Read the model definition and answer for the solid it produces. Units are mm, in the model's axes. A direction names the side the tool comes from. Coordinates: 2 decimals unless noted, no trailing zeros. Order: outer loops, then holes, each group sorted by start corner. A loop starts at its lowest first (then second) coordinate and runs counter-clockwise, first axis right, second up.
```python
from build123d import *

# Parameters (mm, degrees)
SKETCH1_W           = 42
SKETCH1_H           = 67.5
SKETCH1_R           = 3
SKETCH1_R_2         = 2.25
BOSS_EXTRUDE1_DEPTH = 4
SKETCH2_W           = 42
SKETCH2_H           = 3
BOSS_EXTRUDE2_DEPTH = 12
SKETCH3_W           = 42
SKETCH3_H           = 16
SKETCH3_R           = 3
BOSS_EXTRUDE3_DEPTH = 3
CUT_EXTRUDE1_REACH  = 74.479
SKETCH4_R           = 1.6
FILLET1_R           = 4
SKETCH5_W           = 16
SKETCH5_H           = 16
BOSS_EXTRUDE4_DEPTH = 3
FILLET3_R           = 2
FILLET4_R           = 2


with BuildPart() as part:
    # Sketch1 → Boss-Extrude1 (new body)
    with BuildSketch(Plane.XY):
        Rectangle(SKETCH1_W, SKETCH1_H)
        with Locations((-7.5, -24.75)):
            Circle(SKETCH1_R, mode=Mode.SUBTRACT)
        with Locations((1.5, 29.25)):
            Circle(SKETCH1_R_2, mode=Mode.SUBTRACT)
        with Locations((-16.5, 29.25)):
            Circle(SKETCH1_R_2, mode=Mode.SUBTRACT)
        with Locations((1.5, 5.25)):
            Circle(SKETCH1_R_2, mode=Mode.SUBTRACT)
        with Locations((-16.5, 5.25)):
            Circle(SKETCH1_R_2, mode=Mode.SUBTRACT)
    extrude(amount=BOSS_EXTRUDE1_DEPTH)

    # Sketch2 → Boss-Extrude2 (add)
    with BuildSketch(Plane.XY.offset(4)):
        with Locations((0, -32.25)):
            Rectangle(SKETCH2_W, SKETCH2_H)
    extrude(amount=BOSS_EXTRUDE2_DEPTH)

    # Sketch3 → Boss-Extrude3 (add)
    with BuildSketch(Plane.XY.offset(4)):
        with Locations((0, -22.75)):
            Rectangle(SKETCH3_W, SKETCH3_H)
        with Locations((-7.5, -24.75)):
            Circle(SKETCH3_R, mode=Mode.SUBTRACT)
    extrude(amount=BOSS_EXTRUDE3_DEPTH)

    # Sketch4 → Cut-Extrude1 (cut, up to next)
    with BuildSketch(Plane.XZ.offset(33.75), mode=Mode.PRIVATE) as cut_extrude1_sk1:
        with Locations(Location((-15.5, 12.5, 0), (0, 0, 270))):
            Circle(SKETCH4_R)
    cut_extrude1_tool1 = extrude(cut_extrude1_sk1.sketch, amount=-CUT_EXTRUDE1_REACH, mode=Mode.PRIVATE) & part.part
    # Sketch4 → Cut-Extrude1 (cut, up to next)
    with BuildSketch(Plane.XZ.offset(33.75), mode=Mode.PRIVATE) as cut_extrude1_sk2:
        with Locations(Location((15.285724533, 12.5, 0), (0, 0, 270))):
            Circle(SKETCH4_R)
    cut_extrude1_tool2 = extrude(cut_extrude1_sk2.sketch, amount=-CUT_EXTRUDE1_REACH, mode=Mode.PRIVATE) & part.part
    add(cut_extrude1_tool1.solids().sort_by_distance((-15.5, -33.75, 12.5))[0], mode=Mode.SUBTRACT)
    add(cut_extrude1_tool2.solids().sort_by_distance((15.285725, -33.75, 12.5))[0], mode=Mode.SUBTRACT)

    # Fillet1
    # the kernel refuses this fillet: 4 mm, written as the material it adds along each edge
    with BuildSketch(Plane(origin=(-21, -14.75, 4), x_dir=(0, 1, 0), z_dir=(1, 0, 0))) as fillet1_piece_1:
        with BuildLine():
            CenterArc((3.872983346, 4), FILLET1_R, 194.477512186, 75.522487814)
            Line((0, 3), (0, 0))
            Line((0, 0), (3.872983346, 0))
        make_face()
    extrude(amount=42)
    # the kernel refuses this fillet: 4 mm, written as the material it takes off along each edge
    with BuildSketch(Plane(origin=(21, -20.75, 16), x_dir=(0, 0, -1), z_dir=(0, -1, 0)), Plane(origin=(-21, -43.75, 16), x_dir=(0, 0, -1), z_dir=(0, 1, 0))) as fillet1_2_piece_1:
        with BuildLine():
            CenterArc((FILLET1_R, -FILLET1_R), FILLET1_R, 90, 90)
            Line((0, -FILLET1_R), (0, 0))
            Line((0, 0), (FILLET1_R, 0))
        make_face()
    extrude(amount=23, mode=Mode.SUBTRACT)
    with BuildSketch(Plane(origin=(21, 33.75, -10), x_dir=(-1, 0, 0), z_dir=(0, 0, 1))) as fillet1_2_piece_2:
        with BuildLine():
            CenterArc((FILLET1_R, FILLET1_R), FILLET1_R, 180, 90)
            Line((0, FILLET1_R), (0, 0))
            Line((0, 0), (FILLET1_R, 0))
        make_face()
    extrude(amount=24, mode=Mode.SUBTRACT)
    with BuildSketch(Plane(origin=(-21, 33.75, -10), x_dir=(1, 0, 0), z_dir=(0, 0, 1))) as fillet1_2_piece_3:
        with BuildLine():
            CenterArc((FILLET1_R, -FILLET1_R), FILLET1_R, 90, 90)
            Line((0, -FILLET1_R), (0, 0))
            Line((0, 0), (FILLET1_R, 0))
        make_face()
    extrude(amount=24, mode=Mode.SUBTRACT)

    # Sketch5 → Boss-Extrude4 (add)
    with BuildSketch(Plane.XZ.offset(33.75)):
        with Locations((-0.071835854, 8)):
            Rectangle(SKETCH5_W, SKETCH5_H)
    extrude(amount=BOSS_EXTRUDE4_DEPTH)

    # Fillet3
    fillet3_edges = [part.edges().sort_by_distance(p)[0] for p in [
        (-8.071835854, -33.75, 8),
        (7.928164146, -33.75, 8),
    ]]
    fillet(fillet3_edges, radius=FILLET3_R)

    # Fillet4
    fillet4_edges = [part.edges().sort_by_distance(p)[0] for p in [
        (7.928164146, -36.75, 8),
        (-8.071835854, -36.75, 8),
    ]]
    fillet(fillet4_edges, radius=FILLET4_R)


solid = part.part
```
1) A cutting plane is placed at B-B, the plane y = 5.25. Determine the outline of the cut face in (x, z).
A:
outline: (-21, 0) - (-18.75, 0) - (-18.75, 4) - (-21, 4) - close; (-14.25, 0) - (-0.75, 0) - (-0.75, 4) - (-14.25, 4) - close; (3.75, 0) - (21, 0) - (21, 4) - (3.75, 4) - close
2) Straight lines are drawn through the part: line 1 (Y direction, x = 1.5, z = 1.2); line 2 (Y direction, x = -16.5, z = 2.4); line 3 (X direction, y = -32, z = 12.5). For each, find the intervals that lie inside material, in ascending order.
A:
line 1: y = -36.75 to 3, 7.5 to 27, 31.5 to 33.75
line 2: y = -33.75 to 3, 7.5 to 27, 31.5 to 33.75
line 3: x = -20.97 to -17.1, -13.9 to 13.69, 16.89 to 20.97
3) Determine the mould class of faces 4 (the cylindrical face through (16.367, -32.271, 13.679)), 5 (the cylindrical face through (19.859, -32.229, 14.797)), 6 (the cylindrical face through (-8.86, -34.16, 8.11)) for opening direction X: pulls with the +X half, pulls with the -X half, needs draft (parallel to the pull), parting line crosses it, or undercut.
A:
face 4: undercut
face 5: pulls with the +X half
face 6: pulls with the -X half
4) A cutting plane is placed at D-D, the plane z = 1.5. State how many separate pieces and enclosed holes the cut face has, and give its area (3 significant figures).
A:
separate pieces: 1
enclosed holes: 5
area: 2,780 mm2
5) Flat-ended cylindrical pins translate along their axes: pin 1 Ø6 at (x, z) = (-7.5, 7.5) entering from +Y; pin 2 Ø2.5 at (x, z) = (-15.5, 12.5) entering from -Y; pin 3 Ø3.5 at (x, z) = (15.5, 11) entering from -Y; pin 4 Ø6 at (x, y) = (-16.5, 29.25) entering from +Z. Find the tip coordinate at first contact, or state that the pin passes through.
A:
pin 1: stops at y = -12.81
pin 2: passes through
pin 3: stops at y = -33.75
pin 4: stops at z = 4
6) A cutting plane is placed at A-A, the plane y = -24.75. Determine the outline of the cut face in (x, z).
A:
outline: (-21, 0) - (-10.5, 0) - (-10.5, 7) - (-21, 7) - close; (-4.5, 0) - (21, 0) - (21, 7) - (-4.5, 7) - close
7) A cutting plane is placed at C-C, the plane x = -15.5. Determine the outline of the cut face in (y, z).
A:
outline: (-33.75, 0) - (3.23, 0) - (3.23, 4) - (-10.88, 4) arc R4 cw to (-14.75, 7) - (-30.75, 7) - (-30.75, 10.9) - (-33.75, 10.9) - close; (-33.75, 14.1) - (-30.75, 14.1) - (-30.75, 16) - (-33.75, 16) - close; (7.27, 0) - (27.23, 0) - (27.23, 4) - (7.27, 4) - close; (31.27, 0) - (33.75, 0) - (33.75, 4) - (31.27, 4) - close
8) Which of the six approach directions +Z, -Z, +X, -X, +Y, -Y give full straight-line access (tool end or side, diameter ignored) to faces 1 (the flat face through (15, -33.75, 8)), 2 (the flat face through (0, -30.75, 11)), 3 (the flat face through (0, 33.75, 2))?
A:
face 1: +Z, -Z, +X, -Y
face 2: +Z, +X, -X, +Y
face 3: +Z, -Z, +X, -X, +Y
